from build123d import *

# Parameters (mm, degrees)
SKETCH1_W           = 86.8
SKETCH1_H           = 68.4
BOSS_EXTRUDE1_DEPTH = 3
SKETCH2_W           = 10
SKETCH2_H           = 3
BOSS_EXTRUDE2_DEPTH = 20
SKETCH3_W           = 10
SKETCH3_H           = 3
BOSS_EXTRUDE3_DEPTH = 20
SKETCH4_R           = 1
CUT_EXTRUDE1_DEPTH  = 20
SKETCH5_R           = 1.5
CUT_EXTRUDE2_DEPTH  = 20
SKETCH8_R           = 1.5
CUT_EXTRUDE3_DEPTH  = 20
CUT_EXTRUDE4_DEPTH  = 10


with BuildPart() as part:
    # Sketch1 → Boss-Extrude1 (new body)
    with BuildSketch(Plane(origin=(0, 0, 0), x_dir=(1, 0, 0), z_dir=(0, 1, 0))):
        with Locations((43.4, -34.2)):
            Rectangle(SKETCH1_W, SKETCH1_H)
    extrude(amount=BOSS_EXTRUDE1_DEPTH)

    # Sketch2 → Boss-Extrude2 (add)
    with BuildSketch(Plane(origin=(0, 3, 0), x_dir=(1, 0, 0), z_dir=(0, 1, 0))):
        with Locations((5, -66.9)):
            Rectangle(SKETCH2_W, SKETCH2_H)
    extrude(amount=BOSS_EXTRUDE2_DEPTH)

    # Sketch3 → Boss-Extrude3 (add)
    with BuildSketch(Plane(origin=(0, 3, 0), x_dir=(1, 0, 0), z_dir=(0, 1, 0))):
        with Locations((5, -1.5)):
            Rectangle(SKETCH3_W, SKETCH3_H)
    extrude(amount=BOSS_EXTRUDE3_DEPTH)

    # Sketch4 → Cut-Extrude1 (cut)
    with BuildSketch(Plane.XY.offset(68.4)):
        with Locations((5, 13)):
            Circle(SKETCH4_R)
    extrude(amount=-CUT_EXTRUDE1_DEPTH, mode=Mode.SUBTRACT)

    # Sketch5 → Cut-Extrude2 (cut)
    with BuildSketch(Plane.XY.offset(3)):
        with Locations((5, 13)):
            Circle(SKETCH5_R)
    extrude(amount=-CUT_EXTRUDE2_DEPTH, mode=Mode.SUBTRACT)

    # Sketch8 → Cut-Extrude3 (cut)
    with BuildSketch(Plane.XZ):
        with Locations(Location((51.465174946, 53.4, 0), (0, 0, 270))):
            Circle(SKETCH8_R)
        with Locations(Location((51.465174946, 14.730831909, 0), (0, 0, 270))):
            Circle(SKETCH8_R)
    extrude(amount=-CUT_EXTRUDE3_DEPTH, mode=Mode.SUBTRACT)

    # Sketch9 → Cut-Extrude4 (cut)
    with BuildSketch(Plane.XZ):
        with BuildLine():
            Line((56.809330632, 55.9), (57.369330632, 55.9))
            ThreePointArc((57.369330632, 55.9), (59.869330632, 53.4), (57.369330632, 50.9))
            Line((57.369330632, 50.9), (56.809330632, 50.9))
            ThreePointArc((56.809330632, 50.9), (45.565174946, 53.4), (56.809330632, 55.9))
        make_face()
    extrude(amount=-CUT_EXTRUDE4_DEPTH, mode=Mode.SUBTRACT)


solid = part.part
The model under review builds one solid part; all positions refer to its coordinate system, in mm. A direction names the side the tool comes from. Coordinates: 2 decimals unless noted, no trailing zeros. Loops run counter-clockwise (first coordinate to the right, second up) from the corner with the lowest first, then second, coordinate; pieces in that order, holes last.
(1) Consider section B-B, the plane z = 53.4. Give the boundary of the cut face in (x, y), plus the area to 3 significant figures.
Determined:
outline: (0, 0) - (45.57, 0) - (45.57, 3) - (0, 3) - close; (59.87, 0) - (86.8, 0) - (86.8, 3) - (59.87, 3) - close
area: 217 mm2
(2) Consider section D-D, the plane x = 5. Give the boundary of the cut face in (y, z).
Determined:
outline: (0, 0) - (11.5, 0) - (11.5, 3) - (3, 3) - (3, 65.4) - (12, 65.4) - (12, 68.4) - (0, 68.4) - close; (14, 65.4) - (23, 65.4) - (23, 68.4) - (14, 68.4) - close; (14.5, 0) - (23, 0) - (23, 3) - (14.5, 3) - close
(3) Wall thickness on L1, parallel to X at y = 2, z = 53.4; L2, parallel to Y at x = 68.5, z = 45; L3, parallel to Y at x = 5, z = 2.3: over which ranges is each line inside the solid? List them lowest first.
Determined:
L1: x = 0 to 45.57, 59.87 to 86.8
L2: y = 0 to 3
L3: y = 0 to 11.5, 14.5 to 23
(4) Consider section A-A, the plane y = 13. Give the boundary of the cut face in (x, z), plus the area to 3 significant figures.
Determined:
outline: (0, 0) - (3.5, 0) - (3.5, 3) - (0, 3) - close; (0, 65.4) - (4, 65.4) - (4, 68.4) - (0, 68.4) - close; (6, 65.4) - (10, 65.4) - (10, 68.4) - (6, 68.4) - close; (6.5, 0) - (10, 0) - (10, 3) - (6.5, 3) - close
area: 45.0 mm2
(5) Insertion check: P1, Ø2.5, axis at y = 11.5, z = 66.5, coming from the +X side; P2, Ø8, axis at x = 13.5, y = 14, coming from the +Z side; P3, Ø1.8, axis at x = 51.47, z = 14.73, coming from the +Y side; P4, Ø5, axis at x = 45, z = 48.5, coming from the +Y side. Each pin has a flat end and moves straight along its axis. Give the tip position at first contact, or say it passes through.
Determined:
P1: stops at x = 10
P2: stops at z = 68.4
P3: passes through
P4: stops at y = 3
(6) Consider section C-C, the plane y = 18.75. Give the boundary of the cut face in (x, z).
Determined:
outline: (0, 0) - (10, 0) - (10, 3) - (0, 3) - close; (0, 65.4) - (10, 65.4) - (10, 68.4) - (0, 68.4) - close
(7) Tool access review of faces 4 (the flat face through (10, 13, 2)), 5 (the flat face through (7, 13, 3)), 6 (the flat face through (5, 23, 67)), 7 (the cylindrical face through (59.87, 1.48, 53.45)): name each direction out of +Z, -Z, +X, -X, +Y, -Y from which nothing blocks a thin tool from reaching the whole face with its end or side.
Determined:
face 4: +Z, -Z, +X, +Y
face 5: +X, -X, +Y
face 6: +Z, -Z, +X, -X, +Y
face 7: +Y, -Y
(8) Draft analysis for pull direction Y (two halves, no side actions). For faces 1 (the flat face through (0, 2, 37)), 2 (the cylindrical face through (6.386, 12.425, 1.521)), 3 (the flat face through (43, 0, 34)), state which applies: +Y half, -Y half, draft (parallel to the pull), parting line (faces both ways), or undercut.
Determined:
face 1: draft
face 2: undercut
face 3: -Y half
